```python
from build123d import *

# Parameters (mm, degrees)
SKETCH1_R      = 1.5875
SKETCH1_R_2    = 2.032
EXTRUDE1_DEPTH = 6.35


with BuildPart() as part:
    # Sketch1 → Extrude1 (new body)
    with BuildSketch(Plane.XY):
        with BuildLine():
            Line((-198.340264606, 29.708721685), (-122.140264606, 29.708721685))
            add(Edge.make_bspline(
                [(-84.040264606, 44.567721685), (-98.359806002, 44.567721685), (-110.19434592, 29.708721685), (-122.140264606, 29.708721685)],
                knots=[0, 0, 0, 0, 1, 1, 1, 1], degree=3))
            Line((-84.040264606, 44.567721685), (-31.970264606, 44.567721685))
            add(Edge.make_bspline(
                [(-31.970264606, 44.567721685), (-19.845994983, 44.567721685), (-8.482470496, 29.708721685), (6.129735394, 29.708721685)],
                knots=[0, 0, 0, 0, 1, 1, 1, 1], degree=3))
            Line((6.129735394, 29.708721685), (82.329735394, 29.708721685))
            Line((82.329735394, 29.708721685), (82.329735394, 4.816721685))
            Line((82.329735394, 4.816721685), (6.129735394, 4.816721685))
            add(Edge.make_bspline(
                [(-31.970264606, -10.042278315), (-19.845994974, -10.042278315), (-8.148130117, 4.816721685), (6.129735394, 4.816721685)],
                knots=[0, 0, 0, 0, 1, 1, 1, 1], degree=3))
            Line((-31.970264606, -10.042278315), (-84.040264606, -10.042278315))
            add(Edge.make_bspline(
                [(-84.040264606, -10.042278315), (-95.986183291, -10.042278315), (-107.820723209, 4.816721685), (-122.140264606, 4.816721685)],
                knots=[0, 0, 0, 0, 1, 1, 1, 1], degree=3))
            Line((-122.140264606, 4.816721685), (-198.340264606, 4.816721685))
            Line((-198.340264606, 4.816721685), (-198.340264606, 29.708721685))
        make_face()
        with Locations((-80.230264606, 39.487721685)):
            Circle(SKETCH1_R, mode=Mode.SUBTRACT)
        with Locations((-35.780264606, 39.487721685)):
            Circle(SKETCH1_R, mode=Mode.SUBTRACT)
        with Locations((-80.230264606, -4.962278315)):
            Circle(SKETCH1_R, mode=Mode.SUBTRACT)
        with Locations((-35.780264606, -4.962278315)):
            Circle(SKETCH1_R, mode=Mode.SUBTRACT)
        with Locations((79.154735394, 17.262721685)):
            Circle(SKETCH1_R_2, mode=Mode.SUBTRACT)
        with Locations((-195.165264606, 17.262721685)):
            Circle(SKETCH1_R_2, mode=Mode.SUBTRACT)
    extrude(amount=EXTRUDE1_DEPTH)


solid = part.part
```
Part model, mm, in its own coordinate system. A direction names the side the tool comes from. Give positions to 0.01 mm unless a question says otherwise; leave off trailing zeros. Order: outer loops, then holes, each group sorted by start corner. A loop starts at its lowest first (then second) coordinate and runs counter-clockwise, first axis right, second up. Notation, with made-up numbers: M 47.5,63 L 104.5,63 A27 cw 104.5,87 Z; hole C 38,66 d10. An arc over 180 degrees is marked long. Use a Markdown table: item, result. Add a question column.
(1) Drop flat-ended pins along their axis: P1, Ø3, axis at x = -154, z = 3, coming from the +Y side; P2, Ø3, axis at x = 47.5, z = 3.5, coming from the -Y side; P3, Ø3, axis at x = 0, z = 5.5, coming from the +Y side. Give the stop position or say it passes through.
(2) Saw through at B-B, the plane z = 4.25. Give the number of separate pieces and of enclosed holes in the cut face, and give its area (3 significant figures).
(3) 3-axis set-ups, long thin cutter, end or side, ignore diameter. For faces 1 (the face through (44, 29.709, 3)), 2 (the face through (-161, 29.709, 3)), 3 (the face through (45, 4.817, 3)): which of +Z, -Z, +X, -X, +Y, -Y reach the whole face in a straight line?
(4) Saw through at A-A, the plane x = 22. Give the cut face in (y, z), and give its area (3 significant figures).
(5) Probe line 1 along X through (y, z) = (19, 2.25); line 2 along X through (y, z) = (38.5, 4.25); line 3 along Y through (x, z) = (56.5, 3.25). List the from-to ranges inside material, lowest first. Write a range as [from, to].
Answer key:
| question | item | result |
|---|---|---|
| 1 | P1 | y = 29.71 |
| 1 | P2 | y = 4.82 |
| 1 | P3 | y = 30.99 |
| 2 | separate pieces | 1 |
| 2 | enclosed holes | 6 |
| 2 | area | 9,590 mm^2 |
| 3 | face 1 | +Z, -Z, +X, +Y |
| 3 | face 2 | +Z, -Z, -X, +Y |
| 3 | face 3 | +Z, -Z, +X, -Y |
| 4 | outline | M 4.82,0 L 29.71,0 L 29.71,6.35 L 4.82,6.35 Z |
| 4 | area | 158 mm^2 |
| 5 | line 1 | [-198.34, -196.22], [-194.11, 78.1], [80.21, 82.33] |
| 5 | line 2 | [-101.67, -81.47], [-78.99, -37.02], [-34.54, -16.12] |
| 5 | line 3 | [4.82, 29.71] |
